from build123d import *

# Parameters (mm, degrees)
SKETCH_1_R      = 1.45
SKETCH_1_W      = 25
SKETCH_1_H      = 3
SKETCH_1_W_2    = 3
SKETCH_1_H_2    = 25
SKETCH_1_W_3    = 20
SKETCH_1_H_3    = 20
SKETCH_1_W_4    = 30
SKETCH_1_H_4    = 2.9
SKETCH_1_W_5    = 2.9
SKETCH_1_H_5    = 30
EXTRUDE_2_DEPTH = 3


with BuildPart() as part:
    # 草图1 → 凸台-拉伸2 (new body)
    with BuildSketch(Plane.XY):
        with BuildLine():
            Line((104.9, 107.9), (-4.9, 107.9))
            ThreePointArc((-4.9, 107.9), (-7.021320344, 107.021320344), (-7.9, 104.9))
            Line((-7.9, 104.9), (-7.9, -4.9))
            ThreePointArc((-7.9, -4.9), (-7.021320344, -7.021320344), (-4.9, -7.9))
            Line((-4.9, -7.9), (104.9, -7.9))
            ThreePointArc((104.9, -7.9), (107.021320344, -7.021320344), (107.9, -4.9))
            Line((107.9, -4.9), (107.9, 104.9))
            ThreePointArc((107.9, 104.9), (107.021320344, 107.021320344), (104.9, 107.9))
        make_face()
        with Locations((45, 50)):
            Circle(SKETCH_1_R, mode=Mode.SUBTRACT)
        with Locations((55, 50)):
            Circle(SKETCH_1_R, mode=Mode.SUBTRACT)
        with Locations((19.6, -4.4)):
            Rectangle(SKETCH_1_W, SKETCH_1_H, mode=Mode.SUBTRACT)
        with Locations((-4.4, 19.6)):
            Rectangle(SKETCH_1_W_2, SKETCH_1_H_2, mode=Mode.SUBTRACT)
        with Locations((28, 7.5)):
            Rectangle(SKETCH_1_W_3, SKETCH_1_H, mode=Mode.SUBTRACT)
        with Locations((7.5, 28)):
            Rectangle(SKETCH_1_W_2, SKETCH_1_H_3, mode=Mode.SUBTRACT)
        with Locations((50, -1.45)):
            Rectangle(SKETCH_1_W_4, SKETCH_1_H_4, mode=Mode.SUBTRACT)
        with Locations((72, 7.5)):
            Rectangle(SKETCH_1_W_3, SKETCH_1_H, mode=Mode.SUBTRACT)
        with Locations((80.4, -4.4)):
            Rectangle(SKETCH_1_W, SKETCH_1_H, mode=Mode.SUBTRACT)
        with Locations((104.4, 19.6)):
            Rectangle(SKETCH_1_W_2, SKETCH_1_H_2, mode=Mode.SUBTRACT)
        with Locations((92.5, 28)):
            Rectangle(SKETCH_1_W_2, SKETCH_1_H_3, mode=Mode.SUBTRACT)
        with Locations((-1.45, 50)):
            Rectangle(SKETCH_1_W_5, SKETCH_1_H_5, mode=Mode.SUBTRACT)
        with Locations((7.5, 72)):
            Rectangle(SKETCH_1_W_2, SKETCH_1_H_3, mode=Mode.SUBTRACT)
        with Locations((-4.4, 80.4)):
            Rectangle(SKETCH_1_W_2, SKETCH_1_H_2, mode=Mode.SUBTRACT)
        with Locations((19.6, 104.4)):
            Rectangle(SKETCH_1_W, SKETCH_1_H, mode=Mode.SUBTRACT)
        with Locations((28, 92.5)):
            Rectangle(SKETCH_1_W_3, SKETCH_1_H, mode=Mode.SUBTRACT)
        with Locations((80.4, 104.4)):
            Rectangle(SKETCH_1_W, SKETCH_1_H, mode=Mode.SUBTRACT)
        with Locations((101.45, 50)):
            Rectangle(SKETCH_1_W_5, SKETCH_1_H_5, mode=Mode.SUBTRACT)
        with Locations((92.5, 72)):
            Rectangle(SKETCH_1_W_2, SKETCH_1_H_3, mode=Mode.SUBTRACT)
        with Locations((72, 92.5)):
            Rectangle(SKETCH_1_W_3, SKETCH_1_H, mode=Mode.SUBTRACT)
        with Locations((50, 101.45)):
            Rectangle(SKETCH_1_W_4, SKETCH_1_H_4, mode=Mode.SUBTRACT)
        with Locations((104.4, 80.4)):
            Rectangle(SKETCH_1_W_2, SKETCH_1_H_2, mode=Mode.SUBTRACT)
    extrude(amount=EXTRUDE_2_DEPTH)


solid = part.part
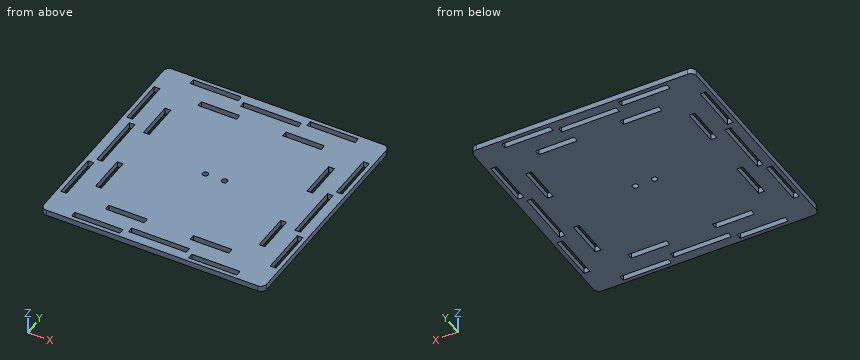
The listing builds one solid part. Answer for the finished solid, in the listing's coordinates (mm). Round coordinates to 2 decimals unless told otherwise and drop trailing zeros. Write each loop counter-clockwise with the first axis right and the second up, starting at its lowest first coordinate (ties: lowest second). Pieces come first, ordered by that corner, then holes. Notation, with made-up numbers: M -4,77.25 L 2,77.25 A16 cw 2,105.25 Z; hole C -32,42 d10. An arc over 180 degrees is marked long. Write each question's results on one line, items separated by ' | '. Start each with the question number.
Item 1: Find section A-A on x = 48.5. Write down the section's boundary in (y, z).
Item 2: Find section B-B on y = 50. Write down the section's boundary in (x, z), and give its area (3 significant figures).
Item 3: Find section D-D on z = 2.05. Give the number of separate pieces and of enclosed holes in the cut face, and give its area (3 significant figures).
Item 4: Find section C-C on x = 74.5. Write down the section's boundary in (y, z), and give its area (3 significant figures).
Item 5: Straight lines are drawn through the part: probe 1 along Y at (x, z) = (90.5, 2.5); probe 2 along X at (y, z) = (91.5, 2); probe 3 along X at (y, z) = (75.5, 2.1). For each, find the intervals that lie inside material, in ascending order.
Answer block:
1) outline: M -7.9,0 L -2.9,0 L -2.9,3 L -7.9,3 Z; M 0,0 L 100,0 L 100,3 L 0,3 Z; M 102.9,0 L 107.9,0 L 107.9,3 L 102.9,3 Z
2) outline: M -7.9,0 L -2.9,0 L -2.9,3 L -7.9,3 Z; M 0,0 L 43.55,0 L 43.55,3 L 0,3 Z; M 46.45,0 L 53.55,0 L 53.55,3 L 46.45,3 Z; M 56.45,0 L 100,0 L 100,3 L 56.45,3 Z; M 102.9,0 L 107.9,0 L 107.9,3 L 102.9,3 Z | area: 313 mm²
3) separate pieces: 1 | enclosed holes: 22 | area: 12,000 mm²
4) outline: M -7.9,0 L -5.9,0 L -5.9,3 L -7.9,3 Z; M -2.9,0 L 6,0 L 6,3 L -2.9,3 Z; M 9,0 L 91,0 L 91,3 L 9,3 Z; M 94,0 L 102.9,0 L 102.9,3 L 94,3 Z; M 105.9,0 L 107.9,0 L 107.9,3 L 105.9,3 Z | area: 311 mm²
5) probe 1: y = -7.9 to -5.9, -2.9 to 102.9, 105.9 to 107.9 | probe 2: x = -7.9 to -5.9, -2.9 to 18, 38 to 62, 82 to 102.9, 105.9 to 107.9 | probe 3: x = -7.9 to -5.9, -2.9 to 6, 9 to 91, 94 to 102.9, 105.9 to 107.9
